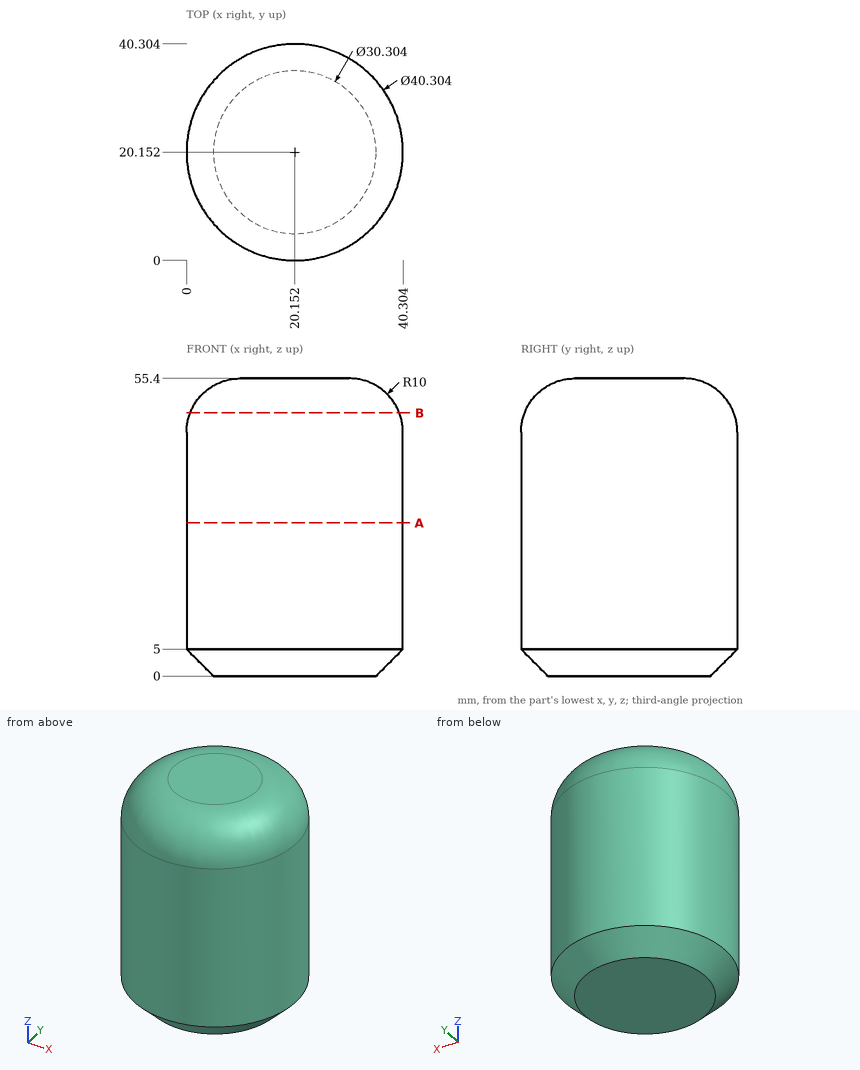
For this review, use the dimensioned drawing (mm, ordinates from the lowest corner) and the shaded views. Coordinates: 2 decimals unless noted, no trailing zeros. Loops run counter-clockwise (first coordinate to the right, second up) from the corner with the lowest first, then second, coordinate; pieces in that order, holes last. Notation, with made-up numbers: (70.5, 21.25) -> (79.5, 21.25) arc R33 cw to (79.5, 57.25) -> close; hole circle Ø6 at (26, 38). An arc over 180 degrees is marked (long way). Use a Markdown table: item, result. Add a question column.
Item 1: Clearance check with flat-ended pins moving along their axes: P1, Ø12, axis at x = 34.5, z = 8, coming from the +Y side; P2, Ø5, axis at x = 19, z = 10, coming from the +Y side; P3, Ø8, axis at y = 31.5, z = 40, coming from the +X side. State where each tip first meets the part, or that it passes through.
Item 2: We need section A-A, the plane z = 28.5. Write out the cut boundary in (x, y).
Item 3: We need section B-B, the plane z = 49. Write out the cut boundary in (x, y).
Item 4: Wall thickness on L1, parallel to X at y = 19.5, z = 39; L2, parallel to X at y = 24, z = 7; L3, parallel to Y at x = 34.5, z = 3.5: over which ranges is each line inside the solid? List them lowest first. Write a range as from..to.
Numbers:
| question | item | result |
|---|---|---|
| 1 | P1 | stops at y = 38.49 |
| 1 | P2 | stops at y = 40.3 |
| 1 | P3 | stops at x = 38.92 |
| 2 | outline | circle Ø40.3 at (20.15, 20.15) |
| 3 | outline | circle Ø38.96 at (20.15, 20.15) |
| 4 | L1 | x = 0.01..40.29 |
| 4 | L2 | x = 0.37..39.93 |
| 4 | L3 | y = 8.23..32.07 |
